```python
from build123d import *

# Parameters (mm, degrees)
SKETCH_R  = 2.1
PAD_DEPTH = 1


with BuildPart() as part:
    # Sketch → Pad (new body)
    with BuildSketch(Plane.XY):
        with BuildLine():
            ThreePointArc((0, 5), (-5, 0), (0, -5))
            Line((0, -5), (140, -5))
            ThreePointArc((140, -5), (145, 0), (140, 5))
            Line((0, 5), (140, 5))
        make_face()
        Circle(SKETCH_R, mode=Mode.SUBTRACT)
        with Locations((10, 0)):
            Circle(SKETCH_R, mode=Mode.SUBTRACT)
        with Locations((20, 0)):
            Circle(SKETCH_R, mode=Mode.SUBTRACT)
        with Locations((30, 0)):
            Circle(SKETCH_R, mode=Mode.SUBTRACT)
        with Locations((40, 0)):
            Circle(SKETCH_R, mode=Mode.SUBTRACT)
        with Locations((50, 0)):
            Circle(SKETCH_R, mode=Mode.SUBTRACT)
        with Locations((60, 0)):
            Circle(SKETCH_R, mode=Mode.SUBTRACT)
        with Locations((70, 0)):
            Circle(SKETCH_R, mode=Mode.SUBTRACT)
        with Locations((80, 0)):
            Circle(SKETCH_R, mode=Mode.SUBTRACT)
        with Locations((90, 0)):
            Circle(SKETCH_R, mode=Mode.SUBTRACT)
        with Locations((100, 0)):
            Circle(SKETCH_R, mode=Mode.SUBTRACT)
        with Locations((110, 0)):
            Circle(SKETCH_R, mode=Mode.SUBTRACT)
        with Locations((120, 0)):
            Circle(SKETCH_R, mode=Mode.SUBTRACT)
        with Locations((130, 0)):
            Circle(SKETCH_R, mode=Mode.SUBTRACT)
        with Locations((140, 0)):
            Circle(SKETCH_R, mode=Mode.SUBTRACT)
    extrude(amount=PAD_DEPTH)


solid = part.part
```
Here's how the part is built. I have some questions about the finished solid (model axes, mm). Coordinates: 2 decimals unless noted, no trailing zeros. Order: outer loops, then holes, each group sorted by start corner. A loop starts at its lowest first (then second) coordinate and runs counter-clockwise, first axis right, second up.
Item 1: If we section it at C-C, the plane y = 3.75: List the corners of the cut face in (x, z) for me.
Response values:
outline: (-3.31, 0) - (143.31, 0) - (143.31, 1) - (-3.31, 1) - close
Item 2: I need wall thicknesses on probe 1 along Y at (x, z) = (140, 0.45); probe 2 along Y at (x, z) = (138.5, 0.7); probe 3 along X at (y, z) = (2.25, 0.95). Which ranges of each line are inside material? Lowest first, please.
Response values:
probe 1: y = -5 to -2.1, 2.1 to 5
probe 2: y = -5 to -1.47, 1.47 to 5
probe 3: x = -4.47 to 144.47
Item 3: Thinking about a two-plate mould opening in X: for faces 1 (the face through (-5, 0.1, 0.5)), 2 (the face through (22.003, 0.631, 0.493)), 3 (the face through (145, -0.1, 0.5)), which applies, pulls with the +X half, pulls with the -X half, needs draft (parallel to the pull), parting line crosses it, or undercut?
Response values:
face 1: pulls with the -X half
face 2: undercut
face 3: pulls with the +X half
Item 4: If we section it at A-A, the plane x = 100: List the corners of the cut face in (y, z) for me.
Response values:
outline: (-5, 0) - (-2.1, 0) - (-2.1, 1) - (-5, 1) - close; (2.1, 0) - (5, 0) - (5, 1) - (2.1, 1) - close
Item 5: If we section it at B-B, the plane z = 0.55: Give the number of separate pieces and of enclosed holes in the cut face, then the cut area to 3 significant figures.
Response values:
separate pieces: 1
enclosed holes: 15
area: 1,270 mm2
